Source: CAD feature listing. Evaluate the final solid. Frame: model axes, mm. Face numbers are marked on the shaded views. A direction names the side the tool comes from. Give positions to 0.01 mm unless a question says otherwise; leave off trailing zeros. Loops run counter-clockwise (first coordinate to the right, second up) from the corner with the lowest first, then second, coordinate; pieces in that order, holes last. Notation, with made-up numbers: M 53,19 L 68,19 A18 ccw 68,44 Z; hole C 17.25,18.25 d4. An arc over 180 degrees is marked long. Answer in a Markdown table with one row per item.
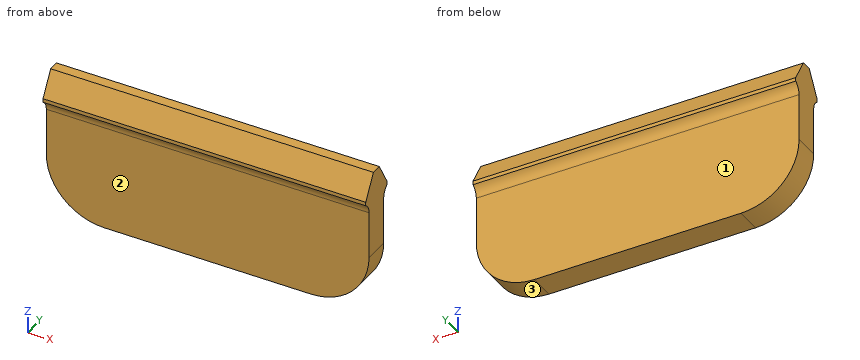
```python
from build123d import *

# Parameters (mm, degrees)
CONNECTION_EXTRUDE_DEPTH = 25
TOP_FILLETS_R            = 4.5
CONNECTION_FILLETS_R     = 1


with BuildPart() as part:
    # Connection Sketch → Connection Extrude (new body)
    with BuildSketch(Plane(origin=(0, 0, 0), x_dir=(0, 0, -1), z_dir=(1, 0, 0))):
        Polygon((0, 1.45), (0, 1), (9, 1), (9, -1), (0, -1), (0, -1.45), (-0.288526329, -1.45), (-2.107179677, -0.4), (-2.107179677, 0.4), (-0.288526329, 1.45), align=None)
    extrude(amount=CONNECTION_EXTRUDE_DEPTH)

    # Top Fillets
    top_fillets_edges = [part.edges().sort_by_distance(p)[0] for p in [
        (0, 0, -9),
        (25, 0, -9),
    ]]
    fillet(top_fillets_edges, radius=TOP_FILLETS_R)

    # Connection Fillets
    # the kernel refuses this fillet: 1 mm, written as the material it adds along each edge
    with BuildSketch(Plane(origin=(0, 1, 0), x_dir=(0, 0, -1), z_dir=(1, 0, 0))) as connection_fillets_piece_1:
        with BuildLine():
            CenterArc((0.835164654, 1), CONNECTION_FILLETS_R, 213.367012969, 56.632987031)
            Line((0, 0.45), (-0.016703293, 0.439))
            ThreePointArc((-0.016703293, 0.439), (-0.02, 0.225), (-0.02, 0))
            Line((-0.02, 0), (0, -0.02))
            Line((0, -0.02), (0.835164654, -0.02))
            Line((0.835164654, -0.02), (0.835164654, 0))
        make_face()
    extrude(amount=25)
    with BuildSketch(Plane(origin=(0, -1, 0), x_dir=(0, 0, -1), z_dir=(1, 0, 0))) as connection_fillets_piece_2:
        with BuildLine():
            CenterArc((0.835164654, -1), CONNECTION_FILLETS_R, 90, 56.632987031)
            Line((0, -0.45), (-0.016703293, -0.439))
            ThreePointArc((-0.016703293, -0.439), (-0.02, -0.225), (-0.02, 0))
            Line((-0.02, 0), (0, 0.02))
            Line((0, 0.02), (0.835164654, 0.02))
            Line((0.835164654, 0.02), (0.835164654, 0))
        make_face()
    extrude(amount=25)


solid = part.part
```
1) Section B-B, the plane z = -1.75. Return loops of the section in (x, y).
Reply:
| item | result |
|---|---|
| outline | M 0,-1 L 25,-1 L 25,1 L 0,1 Z |
2) Section C-C, the plane y = -0.75. Return loops of the section in (x, z).
Reply:
| item | result |
|---|---|
| outline | M 0,-4.5 A4.5 ccw 4.5,-9 L 20.5,-9 A4.5 ccw 25,-4.5 L 25,1.5 L 0,1.5 Z |
3) Material intervals for L1, parallel to Y at x = 14.25, z = -3.25; L2, parallel to Y at x = 15.75, z = -0.25; L3, parallel to Z at x = 12.25, y = 0.55, sorted ascending.
Reply:
| item | result |
|---|---|
| L1 | y = -1 to 1 |
| L2 | y = -1.19 to 1.19 |
| L3 | z = -9 to 1.85 |
4) Set-up query: the marked faces 1, 2 and 3. Return all of +Z, -Z, +X, -X, +Y, -Y with unobstructed straight access to the full face (end or side cutting, diameter ignored); none if empty.
Reply:
| item | result |
|---|---|
| face 1 | -Z, +X, -X, +Y |
| face 2 | -Z, +X, -X, -Y |
| face 3 | -Z, +X, +Y, -Y |
5) Section D-D, the plane x = 2. Return loops of the section in (y, z).
Reply:
| item | result |
|---|---|
| outline | M -1.45,0 A1 cw -1,-0.84 L -1,-8.24 L 1,-8.24 L 1,-0.84 A1 cw 1.45,0 L 1.45,0.29 L 0.4,2.11 L -0.4,2.11 L -1.45,0.29 Z |
6) Section A-A, the plane x = 11.5. Return loops of the section in (y, z), then the cut area to 3 significant figures.
Reply:
| item | result |
|---|---|
| outline | M -1.45,0 A1 cw -1,-0.84 L -1,-9 L 1,-9 L 1,-0.84 A1 cw 1.45,0 L 1.45,0.29 L 0.4,2.11 L -0.4,2.11 L -1.45,0.29 Z |
| area | 22.4 mm² |
7) Pin query (flat end, axial travel): pin 1 Ø4 at (x, z) = (9.5, -4.5) entering from +Y; pin 2 Ø6 at (x, z) = (6.5, -5) entering from -Y. Return the tip coordinate at first contact, or that it passes through.
Reply:
| item | result |
|---|---|
| pin 1 | stops at y = 1 |
| pin 2 | stops at y = -1 |
